Autodesk Inventor part; units mm, degrees
ref_plane "YZ Plane" through (0, 0, 0) normal (1, 0, 0) x (0, 1, 0)
ref_plane "XZ Plane" through (0, 0, 0) normal (0, 1, 0) x (-1, 0, 0)
ref_plane "XY Plane" through (0, 0, 0) normal (0, 0, 1) x (1, 0, 0)
sketch "Sketch1" plane through (0, 0, 0) normal (0, 1, 0) x (-1, 0, 0)
  line L0 (-15.486, -17.1716) -> (12.514, -17.1716)
  line L1 (12.514, 10.8284) -> (-15.486, 10.8284)
  line L2 (-20.486, 10.8284) -> (12.514, 10.8284) construction
  line L3 (-15.486, 5.8284) -> (-15.486, -12.1716)
  line L4 (12.514, 7.8284) -> (12.514, -12.1716)
  line L5 (12.514, -8.1716) -> (12.514, -3.1716)
  line L6 (7.514, -3.1716) -> (7.514, -8.1716)
  line L7 (7.514, -8.1716) -> (12.514, -8.1716)
  line L8 (12.514, 1.8284) -> (12.514, -3.1716)
  line L9 (7.514, -1.1716) -> (7.514, 1.8284)
  line L10 (7.514, 1.8284) -> (12.514, 1.8284)
  line L11 (12.514, -8.1716) -> (12.514, -3.1716)
  line L12 (12.514, -3.1716) -> (12.514, 1.8284)
  line L13 (12.514, 1.8284) -> (12.514, -3.1716)
  line L14 (12.514, -3.1716) -> (12.514, -8.1716)
  line L15 (12.514, -12.1716) -> (12.514, -17.1716)
  line L16 (12.514, 7.8284) -> (12.514, 10.8284)
  line L17 (-1.486, -17.1716) -> (-1.486, 10.8284)
  circle A0 centre (-12.986, -0.6716) radius 1
  line L18 (-10.486, 1.8284) -> (-15.486, 1.8284)
  line L19 (-15.486, 1.8284) -> (-15.486, -3.1716)
  line L20 (-15.486, -3.1716) -> (-15.486, 1.8284)
  line L21 (-15.486, 1.8284) -> (-15.486, -3.1716)
  line L22 (-10.486, -1.1716) -> (-10.486, 1.8284)
  circle A1 centre (-12.986, -5.6716) radius 1.1
  line L23 (-15.486, -8.1716) -> (-15.486, -3.1716)
  line L24 (-15.486, -8.1716) -> (-15.486, -3.1716)
  line L25 (-15.486, -3.1716) -> (-15.486, -8.1716)
  line L26 (-10.486, -3.1716) -> (-10.486, -8.1716)
  line L27 (-10.486, -8.1716) -> (-15.486, -8.1716)
  line L28 (-15.486, -12.1716) -> (-15.486, -17.1716)
  line L29 (-15.486, 7.8284) -> (-15.486, -12.1716)
  line L30 (-15.486, 10.8284) -> (-15.486, -17.1716)
  line L31 (10.014, -5.6716) -> (12.514, -5.6716)
  line L32 (10.014, -0.6716) -> (12.514, -0.6716)
  circle A2 centre (10.014, -5.6716) radius 1
  circle A3 centre (10.014, -0.6716) radius 1.1
  point P0 (0, 0)
  point P1 (10.014, -8.1716)
  point P2 (10.014, 1.8284)
  point P3 (-12.986, 1.8284)
  point P4 (-12.986, -8.1716)
  point P5 (12.514, 1.8284)
  point P6 (-15.486, 1.8284)
  point P7 (12.514, -8.1716)
  dimension "d0" = 5
  dimension "d1" = 2.5
  dimension "d2" = 2.5
  dimension "d3" = 2
  dimension "d4" = 2.2
  dimension "d5" = 2.2
  dimension "d6" = 28
  dimension "d7" = 28
  dimension "d19" = 28
extrude "Extrusion1" add sketch "Sketch1" along normal blind 5
extrude "Extrusion2" add sketch "Sketch1" along normal blind 7 contours A2 | A0
extrude "Extrusion3" add sketch "Sketch1" along normal blind 2.8 contours A3 | A1
sketch "Sketch2" plane through (0, 5, 0) normal (0, 1, 0) x (1, 0, 0)
  line L0 (-12.514, -10.8284) -> (15.486, -10.8284)
  line L1 (1.486, -10.8284) -> (6.986, -10.8284)
  line L2 (6.986, -10.8284) -> (6.986, -6.3284)
  line L3 (6.986, -6.3284) -> (-4.014, -6.3284)
  line L4 (-4.014, -6.3284) -> (-4.014, -10.8284)
  point P0 (0, 0)
  dimension "d14" = 5.5
  dimension "d15" = 4.5
  dimension "d16" = 11
extrude "Extrusion4" cut sketch "Sketch2" against normal blind 0.1
properties part number "TracciaSopra"
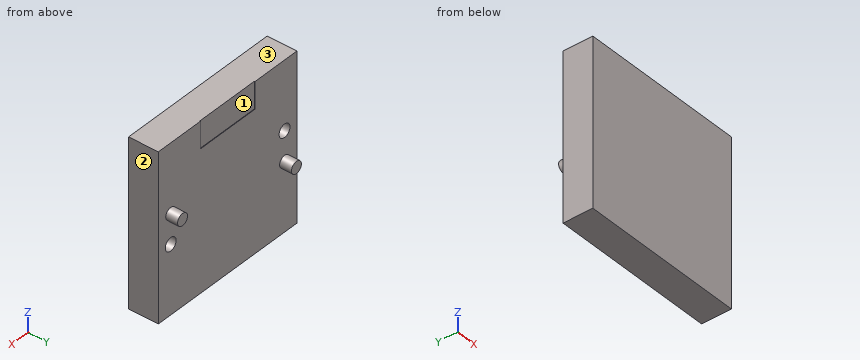
For this review, take the finished solid that the model builds, in its own axes (mm). Face numbers are marked on the shaded views. Coordinates: 2 decimals unless noted, no trailing zeros. Loops run counter-clockwise (first coordinate to the right, second up) from the corner with the lowest first, then second, coordinate; pieces in that order, holes last.
1. Add section B-B, the plane x = 4.75. Give the boundary of the cut face in (y, z).
2. For line 1 (Y direction, x = 3.75, z = -12.75); line 2 (Z direction, x = -10.5, y = 4.5); line 3 (Y direction, x = -9, z = -0.75), list the stretches that pass through material, from the lowest coordinate up.
3. Add section C-C, the plane y = 6.5. Give the boundary of the cut face in (x, z), then the cut area to 3 significant figures.
4. Add section D-D, the plane x = 9. Give the boundary of the cut face in (y, z), then the cut area to 3 significant figures.
5. Mouldability with a two-part tool opening along X and no side actions: class the marked faces 1, 2 and 3 as +X half, -X half, draft (parallel to the pull), parting line (faces both ways), or undercut.
6. Add section A-A, the plane z = 8.25. Give the boundary of the cut face in (x, y).
7. Insertion check: P1, Ø1.5, axis at x = -6, y = 6, coming from the -Z side; P2, Ø1.1, axis at x = 13, z = -6, coming from the +Y side; P3, Ø2, axis at x = 3, z = 8, coming from the +Y side; P4, Ø1.5, axis at x = 3.5, z = 5, coming from the +Y side. Each pin has a flat end and moves straight along its axis. Give the tip position at first contact, or say it passes through.
Result:
1. outline: (0, -17.17) - (5, -17.17) - (5, 6.33) - (4.9, 6.33) - (4.9, 10.83) - (0, 10.83) - close
2. line 1: y = 0 to 5
2. line 2: z = -17.17 to -1.66, 0.32 to 10.83
2. line 3: y = 0 to 2.8
3. outline: circle Ø2 at (-10.01, -5.67); circle Ø2 at (12.99, -0.67)
3. area: 6.28 mm2
4. outline: (0, -17.17) - (5, -17.17) - (5, 10.83) - (0, 10.83) - close
4. area: 140 mm2
5. face 1: undercut
5. face 2: +X half
5. face 3: draft
6. outline: (-12.51, 0) - (15.49, 0) - (15.49, 5) - (6.99, 5) - (6.99, 4.9) - (-4.01, 4.9) - (-4.01, 5) - (-12.51, 5) - close
7. P1: passes through
7. P2: stops at y = 2.8
7. P3: stops at y = 4.9
7. P4: stops at y = 5
